Can you work these out from the model? Positions are in its coordinate system, mm. A direction names the side the tool comes from. Coordinates: 2 decimals unless noted, no trailing zeros. Loops run counter-clockwise (first coordinate to the right, second up) from the corner with the lowest first, then second, coordinate; pieces in that order, holes last.
```python
from build123d import *

# Parameters (mm, degrees)
SKETCH2_W               = 113.195063652
SKETCH2_H               = 64.34953214
BOSS_EXTRUDE1_DEPTH     = 6.35
SKETCH6_W               = 71.546023985
SKETCH6_H               = 19.05
BOSS_EXTRUDE4_DEPTH     = 38.1
SKETCH8_W               = 2.54
SKETCH8_H               = 16.51
CUT_EXTRUDE1_DEPTH      = 63.5
SKETCH11_W              = 97
SKETCH11_H              = 20.82
BOSS_EXTRUDE8_DEPTH     = 6.35
BOSS_EXTRUDE13_DEPTH    = 6.35
BOSS_EXTRUDE14_DEPTH    = 6.35
BOSS_EXTRUDE15_DEPTH    = 6.35
BOSS_EXTRUDE16_DEPTH    = 6.35
SKETCH20_W              = 17.045853961
SKETCH20_H              = 19.05
BOSS_EXTRUDE17_DEPTH    = 38.1
BOSS_EXTRUDE18_REACH    = 134.649
BOSS_EXTRUDE19_DEPTH    = 13.8
SKETCH23_W              = 17.153547373
SKETCH23_H              = 19.05
SKETCH23_W_2            = 8.74383249
SKETCH23_W_3            = 9.06979052
BOSS_EXTRUDE20_DEPTH    = 19.05
SKETCH24_W              = 8.538975884
SKETCH24_H              = 2.032
SKETCH24_W_2            = 6.156345993
CUT_EXTRUDE2_DEPTH      = 15.748
SKETCH25_W              = 6.404810212
SKETCH25_H              = 2.032
CUT_EXTRUDE3_DEPTH      = 153.153507472
SKETCH26_W              = 28.603496075
SKETCH26_H              = 19.05
BOSS_EXTRUDE21_DEPTH    = 7.085056153
BOSS_EXTRUDE22_DEPTH    = 6.35
SKETCH30_W              = 2.54
SKETCH30_H              = 54.505544918
CUT_EXTRUDE4_DEPTH      = 77.978
CUT_EXTRUDE4_DEPTH_BACK = 2.905744
SKETCH32_W              = 7.257489736
SKETCH32_H              = 15.118119189
CUT_EXTRUDE5_DEPTH      = 21.59


with BuildPart() as part:
    # Sketch2 → Boss-Extrude1 (new body)
    with BuildSketch(Plane.XY):
        with Locations((-1.348571368, 4.519536632)):
            Rectangle(SKETCH2_W, SKETCH2_H)
    extrude(amount=BOSS_EXTRUDE1_DEPTH)

    # Sketch6 → Boss-Extrude4 (add)
    with BuildSketch(Plane.XY.offset(6.35)):
        with Locations((19.475948466, 46.219302702)):
            Rectangle(SKETCH6_W, SKETCH6_H)
        with Locations((19.475948466, -37.180229438)):
            Rectangle(SKETCH6_W, SKETCH6_H)
    extrude(amount=-BOSS_EXTRUDE4_DEPTH)

    # Sketch8 → Cut-Extrude1 (cut)
    with BuildSketch(Plane.ZY.offset(16.297063527)):
        with Locations((-24.13, 44.949302702)):
            Rectangle(SKETCH8_W, SKETCH8_H)
        with Locations((-24.13, -35.910229438)):
            Rectangle(SKETCH8_W, SKETCH8_H)
    extrude(amount=-CUT_EXTRUDE1_DEPTH, mode=Mode.SUBTRACT)

    # Sketch11 → Boss-Extrude8 (add)
    with BuildSketch(Plane.XY.offset(6.35)):
        with Locations((-64.797063527, 47.104302702)):
            Rectangle(SKETCH11_W, SKETCH11_H)
        with Locations((-64.797063527, -38.065229438)):
            Rectangle(SKETCH11_W, SKETCH11_H)
    extrude(amount=-BOSS_EXTRUDE8_DEPTH)

    # Sketch16 → Boss-Extrude13 (add)
    with BuildSketch(Plane(origin=(0, 0, 0), x_dir=(-1, 0, 0), z_dir=(0, 0, -1))):
        with BuildLine():
            Line((16.297063527, 51.782302702), (21.12307027, 51.782302702))
            ThreePointArc((21.12307027, 51.782302702), (23.15507027, 49.75029933), (21.123063527, 47.718302702))
            Line((21.123063527, 47.718302702), (16.297063527, 47.718302702))
            Line((16.297063527, 47.718302702), (16.297063527, 51.782302702))
        make_face()
    extrude(amount=BOSS_EXTRUDE13_DEPTH)

    # Sketch17 → Boss-Extrude14 (add)
    with BuildSketch(Plane(origin=(0, 0, 0), x_dir=(-1, 0, 0), z_dir=(0, 0, -1))):
        with BuildLine():
            Line((16.297063527, -38.607229438), (21.12307027, -38.607229438))
            ThreePointArc((21.12307027, -38.607229438), (23.15507027, -40.63923281), (21.123063527, -42.671229438))
            Line((21.123063527, -42.671229438), (16.297063527, -42.671229438))
            Line((16.297063527, -42.671229438), (16.297063527, -38.607229438))
        make_face()
    extrude(amount=BOSS_EXTRUDE14_DEPTH)

    # Sketch18 → Boss-Extrude15 (add)
    with BuildSketch(Plane(origin=(0, 0, 0), x_dir=(-1, 0, 0), z_dir=(0, 0, -1))):
        with BuildLine():
            Line((113.297063527, 51.782302702), (108.696564152, 51.782302702))
            ThreePointArc((108.696564152, 51.782302702), (106.664564152, 49.750302702), (108.696564152, 47.718302702))
            Line((108.696564152, 47.718302702), (113.297063527, 47.718302702))
            Line((113.297063527, 47.718302702), (113.297063527, 51.782302702))
        make_face()
    extrude(amount=BOSS_EXTRUDE15_DEPTH)

    # Sketch19 → Boss-Extrude16 (add)
    with BuildSketch(Plane(origin=(0, 0, 0), x_dir=(-1, 0, 0), z_dir=(0, 0, -1))):
        with BuildLine():
            Line((113.297063527, -38.607229438), (108.696564152, -38.607229438))
            ThreePointArc((108.696564152, -38.607229438), (106.664564152, -40.639229438), (108.696564152, -42.671229438))
            Line((108.696564152, -42.671229438), (113.297063527, -42.671229438))
            Line((113.297063527, -42.671229438), (113.297063527, -38.607229438))
        make_face()
    extrude(amount=BOSS_EXTRUDE16_DEPTH)

    # Sketch20 → Boss-Extrude17 (add)
    with BuildSketch(Plane(origin=(0, 0, -31.75), x_dir=(-1, 0, 0), z_dir=(0, 0, -1))):
        with Locations((-63.771887439, -37.180229438)):
            Rectangle(SKETCH20_W, SKETCH20_H)
    extrude(amount=-BOSS_EXTRUDE17_DEPTH)

    # Boss-Extrude18: up to this plane
    boss_extrude18_end = Plane(origin=(55.616772372, -37.189415156, -54.156592283), z_dir=(-0.06975647374413249, 0, -0.9975640502598238))
    # Sketch21 → Boss-Extrude18 (add, up to the surface)
    with BuildSketch(Plane(origin=(0, 0, -31.75), x_dir=(-1, 0, 0), z_dir=(0, 0, -1)), mode=Mode.PRIVATE) as boss_extrude18_sk1:
        Polygon((-55.445234397, -27.655229438), (-55.574918488, -30.289415156), (-67.745199901, -30.289415156), (-67.745199901, -44.089415156), (-55.574918488, -44.089415156), (-55.574918488, -46.705229438), (-72.294814419, -46.705229438), (-72.294814419, -27.655229438), align=None)
    boss_extrude18_tool1 = split(extrude(boss_extrude18_sk1.sketch, amount=BOSS_EXTRUDE18_REACH, mode=Mode.PRIVATE), bisect_by=boss_extrude18_end, keep=Keep.BOTH, mode=Mode.PRIVATE)
    add(boss_extrude18_tool1.solids().sort_by_distance((55.764094, -28.959817, -31.75))[0])

    # Sketch22 → Boss-Extrude19 (add)
    with BuildSketch(Plane.XZ.offset(30.289415156)):
        Polygon((55.574918488, -47.316538406), (56.82562534, -47.316538406), (56.82562534, -54.153665574), (56.819539444, -54.24069795), (55.574918488, -54.153665574), align=None)
    extrude(amount=BOSS_EXTRUDE19_DEPTH)

    # Sketch23 → Boss-Extrude20 (add)
    with BuildSketch(Plane(origin=(0, 0, -31.75), x_dir=(-1, 0, 0), z_dir=(0, 0, -1))):
        with Locations((7.720289841, -37.180229438)):
            Rectangle(SKETCH23_W, SKETCH23_H)
        with Locations((-50.877044213, 46.219302702)):
            Rectangle(SKETCH23_W_2, SKETCH23_H)
        with Locations((-51.040023228, -37.180229438)):
            Rectangle(SKETCH23_W_3, SKETCH23_H)
    extrude(amount=BOSS_EXTRUDE20_DEPTH)

    # Sketch24 → Cut-Extrude2 (cut)
    with BuildSketch(Plane(origin=(0, -27.655229438, 0), x_dir=(1, 0, 0), z_dir=(0, 1, 0))):
        with Locations((-3.413004096, 45.974)):
            Rectangle(SKETCH24_W, SKETCH24_H)
        with Locations((49.583300965, 45.974)):
            Rectangle(SKETCH24_W_2, SKETCH24_H)
    extrude(amount=-CUT_EXTRUDE2_DEPTH, mode=Mode.SUBTRACT)

    # Sketch25 → Cut-Extrude3 (cut, through all)
    with BuildSketch(Plane.XZ.offset(-36.694302702)):
        with Locations((49.707533074, -45.974)):
            Rectangle(SKETCH25_W, SKETCH25_H)
    extrude(amount=-CUT_EXTRUDE3_DEPTH, mode=Mode.SUBTRACT)

    # Sketch26 → Boss-Extrude21 (add)
    with BuildSketch(Plane(origin=(0, 0, -31.75), x_dir=(-1, 0, 0), z_dir=(0, 0, -1))):
        with Locations((-28.33506354, 46.219302702)):
            Rectangle(SKETCH26_W, SKETCH26_H)
    extrude(amount=BOSS_EXTRUDE21_DEPTH)

    # Sketch27 → Boss-Extrude22 (add)
    with BuildSketch(Plane(origin=(0, 0, 0), x_dir=(-1, 0, 0), z_dir=(0, 0, -1))):
        Polygon((-55.248960458, 36.694302702), (-47.14593274, 36.694302702), (-47.14593274, 36.56022062), (27.224261785, 36.56022062), (27.224261785, 29.827699057), (-47.14593274, 29.827699057), (-47.14593274, -22.106759253), (30.255968743, -22.106759253), (30.255968743, -27.655229438), (-47.14593274, -27.655229438), (-55.248960458, -27.655229438), align=None)
    extrude(amount=BOSS_EXTRUDE22_DEPTH)

    # Sketch30 → Cut-Extrude4 (cut, two sides)
    with BuildSketch(Plane.ZY.offset(-47.14593274)) as cut_extrude4_sk:
        with Locations((-3.17615729, 3.825374341)):
            Rectangle(SKETCH30_W, SKETCH30_H)
    extrude(amount=CUT_EXTRUDE4_DEPTH, mode=Mode.SUBTRACT)
    extrude(cut_extrude4_sk.sketch, amount=-CUT_EXTRUDE4_DEPTH_BACK, mode=Mode.SUBTRACT)

    # Sketch32 → Cut-Extrude5 (cut)
    with BuildSketch(Plane.ZY.offset(-46.505127968)):
        with Locations((-35.378744868, -37.488489942)):
            Rectangle(SKETCH32_W, SKETCH32_H)
    extrude(amount=-CUT_EXTRUDE5_DEPTH, mode=Mode.SUBTRACT)


solid = part.part
```
Item 1: I'm going to push flat-ended pins straight in: P1, Ø3, axis at x = -57, y = 30.5, coming from the -Z side; P2, Ø1.5, axis at x = 25, z = -5, coming from the +Y side; P3, Ø1, axis at x = -58.5, y = 1.5, coming from the +Z side; P4, Ø2.5, axis at x = -18, z = -2, coming from the -Y side. Where does each tip first touch, or does it pass through?
Results are:
P1: stops at z = 0
P2: stops at y = 55.74
P3: passes through
P4: stops at y = -42.67
Item 2: Suppose I cut it at D-D, the plane y = 8.5. Please give me the cut outline in (x, z).
Results are:
outline: (-57.95, 0) - (47.15, 0) - (47.15, -1.91) - (50.05, -1.91) - (50.05, -4.45) - (47.15, -4.45) - (47.15, -6.35) - (55.25, -6.35) - (55.25, 6.35) - (-57.95, 6.35) - close
Item 3: On a 3-axis mill with a long thin cutter (end or side, diameter ignored), from which of +Z, -Z, +X, -X, +Y, -Y can I reach the whole of each face in a straight line? I mean faces 1 (the face through (55.249, 32, -3)), 2 (the face through (50, 46, -46.99)), 3 (the face through (46.505, -37, -43)). Say none if no direction works.
Results are:
face 1: +Z, -Z, +X, +Y
face 2: -X, +Y
face 3: -Z, +Y, -Y
Item 4: Suppose I cut it at A-A, the plane z = -36. Please give me the cut outline in (x, y).
Results are:
outline: (-16.3, -46.71) - (0.86, -46.71) - (0.86, -27.66) - (-16.3, -27.66) - close; (14.03, 36.69) - (42.64, 36.69) - (42.64, 55.74) - (14.03, 55.74) - close; (46.51, -46.71) - (72.29, -46.71) - (72.29, -27.66) - (46.51, -27.66) - (46.51, -29.93) - (68.1, -29.93) - (68.1, -45.05) - (46.51, -45.05) - close; (46.51, 36.69) - (55.25, 36.69) - (55.25, 55.74) - (46.51, 55.74) - close
Item 5: Suppose I cut it at B-B, the plane x = -67. Please give me the cut outline in (y, z), plus the area to 3 significant figures.
Results are:
outline: (-48.48, 0) - (-27.66, 0) - (-27.66, 6.35) - (-48.48, 6.35) - close; (36.69, 0) - (57.51, 0) - (57.51, 6.35) - (36.69, 6.35) - close
area: 264 mm2
Item 6: We'd pull the mould along Y, two halves only. Please class faces 4 (the face through (-65, -48.475, 3)), 5 (the face through (57, -45.048, -35)), 6 (the face through (-113.297, 47, 2)): +Y half, -Y half, draft (parallel to the pull), parting line (faces both ways), or undercut.
Results are:
face 4: -Y half
face 5: undercut
face 6: draft
Item 7: Suppose I cut it at C-C, the plane z = -16. Please give me the cut outline in (x, y), plus the area to 3 significant figures.
Results are:
outline: (-16.3, -46.71) - (72.29, -46.71) - (72.29, -27.66) - (-16.3, -27.66) - close; (-16.3, 36.69) - (55.25, 36.69) - (55.25, 55.74) - (-16.3, 55.74) - close
area: 3,050 mm2
Item 8: I need wall thicknesses on line 1 along Y through (x, z) = (52.5, -35); line 2 along Z through (x, y) = (55, -31.5); line 3 along Z through (x, y) = (31.5, -36). Which ranges of each line are inside material? Lowest first, please.
Results are:
line 1: y = -46.71 to -45.05, -29.93 to -27.66, 36.69 to 55.74
line 2: z = -50.8 to -39.01, -31.75 to 6.35
line 3: z = -31.75 to -25.4, -22.86 to 6.35
